Input: part model. Units: mm. Frame: model coordinates. Face numbers are marked on the shaded views. A direction names the side the tool comes from. Coordinates: 2 decimals unless noted, no trailing zeros. Loops run counter-clockwise (first coordinate to the right, second up) from the corner with the lowest first, then second, coordinate; pieces in that order, holes last.
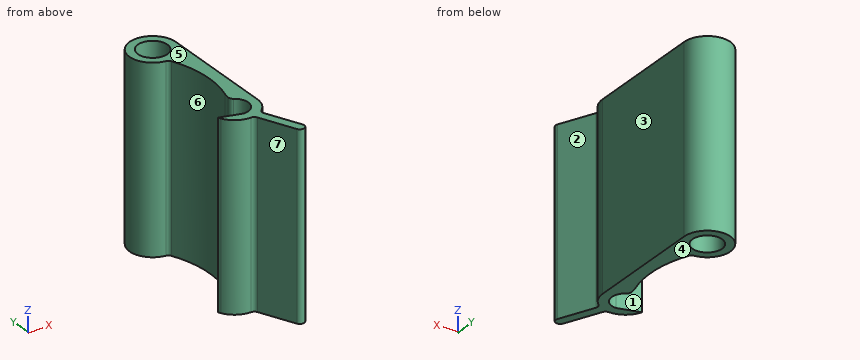
```python
from build123d import *

# Parameters (mm, degrees)
SKETCH1_R           = 2.5
SKETCH1_R_2         = 1.6
BOSS_EXTRUDE1_DEPTH = 19.8
FILLET1_R           = 0.5
BOSS_EXTRUDE2_START = -19.8
BOSS_EXTRUDE2_DEPTH = 19.8
FILLET2_R           = 0.5


with BuildPart() as part:
    # Sketch1 → Boss-Extrude1 (new body)
    # profile 1 of 5: a face of its own
    with BuildSketch(Plane.XY):
        Circle(SKETCH1_R)
        with Locations(Location((0, 0, 0), (0, 0, 180))):
            Circle(SKETCH1_R_2, mode=Mode.SUBTRACT)
    # profile 2 of 5: a face of its own
    with BuildSketch(Plane.XY):
        with BuildLine():
            Line((2.5, -13), (2.5, 0))
            ThreePointArc((2.5, 0), (1.767766953, -1.767766953), (0, -2.5))
            ThreePointArc((0, -2.5), (1.095258289, -6.480732801), (0.645816542, -10.584855906))
            ThreePointArc((0.645816542, -10.584855906), (1.98299538, -11.477590948), (2.5, -13))
        make_face()
    # profile 3 of 5: a face of its own
    with BuildSketch(Plane.XY):
        with BuildLine():
            ThreePointArc((-2.228856339, -14.132342448), (0.582176585, -15.431269303), (2.5, -13))
            ThreePointArc((2.5, -13), (1.98299538, -11.477590948), (0.645816542, -10.584855906))
            Line((0.645816542, -10.584855906), (0.481752062, -11.579466667))
            ThreePointArc((0.481752062, -11.579466667), (1.48, -13.244131112), (0, -14.5))
            ThreePointArc((0, -14.5), (-0.244131112, -14.48), (-0.481752062, -14.420533333))
            Line((-0.481752062, -14.420533333), (-2.228856339, -14.132342448))
        make_face()
    # profile 4 of 5: a face of its own
    with BuildSketch(Plane.XY):
        with BuildLine():
            Line((0, -14.5), (-0.481752062, -14.420533333))
            ThreePointArc((-0.481752062, -14.420533333), (-0.244131112, -14.48), (0, -14.5))
        make_face()
    # profile 5 of 5: a face of its own
    with BuildSketch(Plane.XY):
        with BuildLine():
            ThreePointArc((-2.34950307, -13.854304), (-2.293397058, -13.995153222), (-2.228856339, -14.132342448))
            Line((-2.228856339, -14.132342448), (-0.481752062, -14.420533333))
            Line((-0.481752062, -14.420533333), (0, -14.5))
            Line((0, -14.5), (-2.34950307, -13.854304))
        make_face()
    extrude(amount=BOSS_EXTRUDE1_DEPTH)

    # Fillet1
    fillet1_edges = [part.edges().sort_by_distance(p)[0] for p in [
        (0.481752062, -11.579466667, 9.9),
        (0, -2.5, 9.9),
    ]]
    fillet(fillet1_edges, radius=FILLET1_R)

    # Sketch2 → Boss-Extrude2 (add)
    with BuildSketch(Plane.XY.offset(19.8).offset(BOSS_EXTRUDE2_START)):
        with BuildLine():
            Line((3.400304681, -19.609307967), (1.36493731, -15.094503793))
            ThreePointArc((1.36493731, -15.094503793), (0.917921591, -15.325385979), (0.433729366, -15.462088308))
            Line((0.433729366, -15.462088308), (2.488663388, -20.020294772))
            Line((2.488663388, -20.020294772), (3.400304681, -19.609307967))
        make_face()
    extrude(amount=BOSS_EXTRUDE2_DEPTH)

    # Fillet2
    fillet2_edges = [part.edges().sort_by_distance(p)[0] for p in [
        (0.433729366, -15.462088308, 9.9),
        (1.36493731, -15.094503793, 9.9),
        (3.400304681, -19.609307967, 9.9),
        (2.488663388, -20.020294772, 9.9),
    ]]
    fillet(fillet2_edges, radius=FILLET2_R - 0.0001)  # a hair under: the kernel refuses the full size


solid = part.part
```
Item 1: Contact query for flat-ended pins moving along their axis: P1, Ø10.5, axis at y = -5, z = 9.5, coming from the +X side; P2, Ø4, axis at y = -6, z = 10, coming from the -X side. Output: stop coordinate, or through.
Result:
P1: stops at x = 2.5
P2: stops at x = 0.61
Item 2: Mould query, pull axis Y, two halves, no side actions, for the marked faces 5, 6 and 7. Classes: +Y half, -Y half, draft (parallel to the pull), parting line (faces both ways), or undercut.
Result:
face 5: draft
face 6: undercut
face 7: -Y half
Item 3: Section query B-B (y = -3.5). Output: boundary loops of the cut face in (x, z), then the cut area to 3 significant figures.
Result:
outline: (0.43, 0) - (2.5, 0) - (2.5, 19.8) - (0.43, 19.8) - close
area: 40.9 mm2
Item 4: Line query: L1, parallel to Y at x = -0.25, z = 13; L2, parallel to Y at x = -0.65, z = 12.25; L3, parallel to X at y = 1.25, z = 18. Output: solid intervals per line, ascending.
Result:
L1: y = -15.49 to -14.43, -2.49 to -1.58, 1.58 to 2.49
L2: y = -15.41 to -14.32, -2.41 to -1.46, 1.46 to 2.41
L3: x = -2.17 to -1, 1 to 2.17
Item 5: Reachability of the marked faces 1, 2, 3 and 4 from +Z, -Z, +X, -X, +Y, -Y: full face, straight path, thin tool, end or side. Return the list, or none.
Result:
face 1: +Z, -Z
face 2: +Z, -Z, +X
face 3: +Z, -Z, +X, +Y
face 4: -Z, +X, -X, +Y, -Y
Item 6: Section query A-A (x = -1.35). Output: boundary loops of the cut face in (y, z), then the cut area to 3 significant figures.
Result:
outline: (-15.1, 0) - (-14.13, 0) - (-14.13, 19.8) - (-15.1, 19.8) - close; (-2.1, 0) - (-0.86, 0) - (-0.86, 19.8) - (-2.1, 19.8) - close; (0.86, 0) - (2.1, 0) - (2.1, 19.8) - (0.86, 19.8) - close
area: 68.6 mm2
Item 7: Section query C-C (y = -16.75). Output: boundary loops of the cut face in (x, z).
Result:
outline: (1.01, 0) - (2.11, 0) - (2.11, 19.8) - (1.01, 19.8) - close
